```python
from build123d import *

# Parameters (mm, degrees)
F1_DEPTH = 3
F2_SCALE = 1.5


with BuildPart() as f1:
    # F0 (on Top) → F1 (new body)
    with BuildSketch(Plane.XY):
        with BuildLine():
            Line((-2.279421823, 14.1675013068), (-21.849297046, -8.7031758937))
            ThreePointArc((-21.849297046, -8.7031758937), (-21.8731761415, -10.6250020098), (-19.9867063483, -10.9927214012))
            Line((-19.9867063483, -10.9927214012), (0, 0))
            Line((0, 0), (19.9867063483, -10.9927214012))
            ThreePointArc((19.9867063483, -10.9927214012), (21.8731761415, -10.6250020098), (21.849297046, -8.7031758937))
            Line((21.849297046, -8.7031758937), (2.279421823, 14.1675013068))
            ThreePointArc((2.279421823, 14.1675013068), (0, 15.2170561903), (-2.279421823, 14.1675013068))
        make_face()
    extrude(amount=-F1_DEPTH)


with BuildPart() as f1_1:
    # F2: moved
    add(f1.part.scale(F2_SCALE))


solid = f1_1.part
```
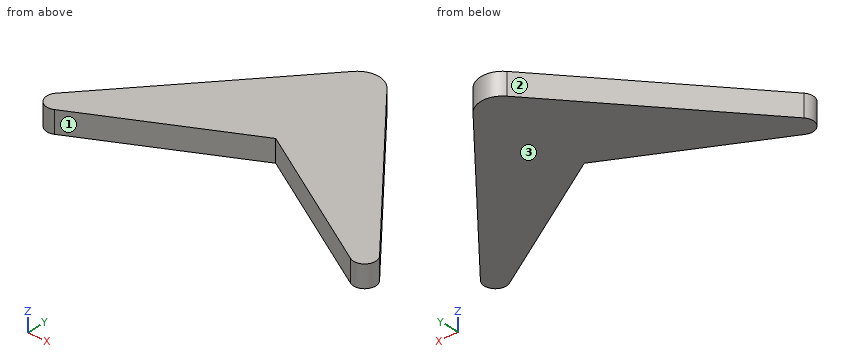
Here's how the part is built. I have some questions about the finished solid (model axes, mm). Face numbers are marked on the shaded views. Coordinates: 2 decimals unless noted, no trailing zeros. Write each loop counter-clockwise with the first axis right and the second up, starting at its lowest first coordinate (ties: lowest second). Pieces come first, ordered by that corner, then holes. Notation, with made-up numbers: M 33.25,88.5 L 65.25,88.5 A10 ccw 65.25,97.5 Z; hole C -12.5,-26 d4. An arc over 180 degrees is marked long. Answer as CSV lines item,"result". Start each with the question number.
Q1. Suppose I cut it at C-C, the plane x = 12. List the corners of the cut face in (y, z) for me.
Q2. Suppose I cut it at A-A, the plane y = -1.5. List the corners of the cut face in (x, z) for me.
Q3. Suppose I cut it at B-B, the plane z = -2.85. List the corners of the cut face in (x, y) for me, then the cut area to 3 significant figures.
Q4. If we mould it in two halves opening along X, with no side actions, what happens to the marked faces 1, 2 and 3? For each: pulls with the +X half, pulls with the -X half, needs draft (parallel to the pull), parting line crosses it, or undercut.
Q5. I need wall thicknesses on probe 1 along X at (y, z) = (-6.5, -3.7); probe 2 along X at (y, z) = (-3.5, -4.2); probe 3 along Y at (x, z) = (16.5, -2.8). Which ranges of each line are inside material? Lowest first, please. Write a range as [from, to].
Q6. Suppose I cut it at D-D, the plane y = 7. List the corners of the cut face in (x, z) for me.
Q7. Will these pins go through, and if not, where does the flat tip stop? pin 1 Ø1 at (x, y) = (-17, -10) entering from -Z; pin 2 Ø1.5 at (y, z) = (-12, -4) entering from -X; pin 3 Ø2 at (x, z) = (-15, -0.5) entering from +Y.
Entries:
1,outline,"M -6.6,-4.5 L 11.22,-4.5 L 11.22,0 L -6.6,0 Z"
2,outline,"M -22.89,-4.5 L -2.73,-4.5 L -2.73,0 L -22.89,0 Z; M 2.73,-4.5 L 22.89,-4.5 L 22.89,0 L 2.73,0 Z"
3,outline,"M -32.77,-13.05 A2.25 ccw -29.98,-16.49 L 0,0 L 29.98,-16.49 A2.25 ccw 32.77,-13.05 L 3.42,21.25 A4.5 ccw -3.42,21.25 Z"
3,area,"983 mm²"
4,face 1,"undercut"
4,face 2,"pulls with the -X half"
4,face 3,"needs draft"
5,probe 1,"x = [-27.17, -11.82], [11.82, 27.17]"
5,probe 2,"x = [-24.6, -6.36], [6.36, 24.6]"
5,probe 3,"y = [-9.08, 5.96]"
6,outline,"M -15.61,-4.5 L 15.61,-4.5 L 15.61,0 L -15.61,0 Z"
7,pin 1,"passes through"
7,pin 2,"stops at x = -32.51"
7,pin 3,"stops at y = 8.89"
